Model file for the job. Use its own axes, mm. Round coordinates to 2 decimals unless told otherwise and drop trailing zeros. Loops run counter-clockwise (first coordinate to the right, second up) from the corner with the lowest first, then second, coordinate; pieces in that order, holes last. Notation, with made-up numbers: M 32.25,69 L 50.25,69 A26 cw 50.25,91 Z; hole C 60.25,-6.5 d8. An arc over 180 degrees is marked long. Use a Markdown table: item, result. Add a question column.
Item 1: Saw through at C-C on z = 0.6. Write the cut outline in (x, y).
Item 2: Saw through at B-B on x = 63. Write the cut outline in (y, z).
Item 3: Wall check: L1, parallel to X at y = 52.5, z = 0.1; L2, parallel to Y at x = 63, z = 0.7; L3, parallel to Y at x = -4, z = 0.45. Give the ranges that are in metal, low to high. Write a range as from..to.
Item 4: Saw through at D-D on x = 13. Write the cut outline in (y, z).
Item 5: Saw through at A-A on y = 55. Write the cut outline in (x, z), then the cut area to 3 significant figures.
```python
from build123d import *

# Parameters (mm, degrees)
F0_W     = 136
F0_H     = 120
F1_DEPTH = 1
F2_W     = 116
F2_H     = 10
F3_DEPTH = 1
F4_R     = 1.5
F5_DEPTH = 1


with BuildPart() as f1:
    # F0 (on Top) → F1 (new body)
    with BuildSketch(Plane.XY):
        Rectangle(F0_W, F0_H)
    extrude(amount=F1_DEPTH)

    # F2 (on face) → F3 (cut, through all)
    with BuildSketch(Plane.XY.offset(1)):
        Polygon((58, 60), (-58, 60), (-58, 50), (-45, 50), (-45, 40), (0, 40), (45, 40), (45, 50), (58, 50), align=None)
        with Locations((0, -55)):
            Rectangle(F2_W, F2_H)
    extrude(amount=-F3_DEPTH, mode=Mode.SUBTRACT)

    # F4 (on face) → F5 (cut, through all)
    with BuildSketch(Plane.XY.offset(1)):
        with Locations((-63, 55)):
            Circle(F4_R)
        with Locations((63, 55)):
            Circle(F4_R)
    extrude(amount=-F5_DEPTH, mode=Mode.SUBTRACT)


solid = f1.part
```
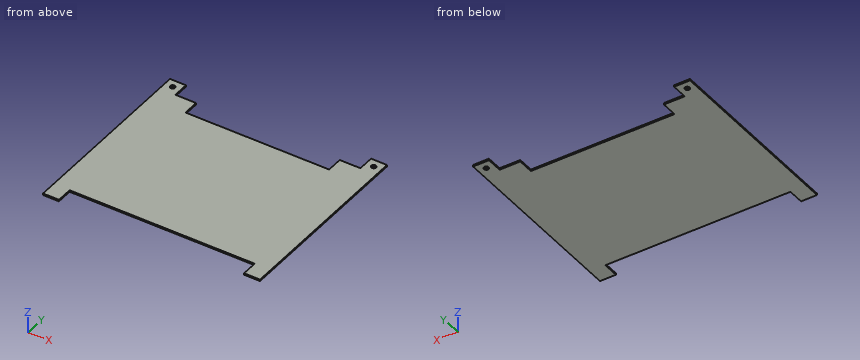
Entries:
| question | item | result |
|---|---|---|
| 1 | outline | M -68,-60 L -58,-60 L -58,-50 L 58,-50 L 58,-60 L 68,-60 L 68,60 L 58,60 L 58,50 L 45,50 L 45,40 L -45,40 L -45,50 L -58,50 L -58,60 L -68,60 Z; hole C -63,55 d3; hole C 63,55 d3 |
| 2 | outline | M -60,0 L 53.5,0 L 53.5,1 L -60,1 Z; M 56.5,0 L 60,0 L 60,1 L 56.5,1 Z |
| 3 | L1 | -68..-58, 58..68 |
| 3 | L2 | -60..53.5, 56.5..60 |
| 3 | L3 | -50..40 |
| 4 | outline | M -50,0 L 40,0 L 40,1 L -50,1 Z |
| 5 | outline | M -68,0 L -64.5,0 L -64.5,1 L -68,1 Z; M -61.5,0 L -58,0 L -58,1 L -61.5,1 Z; M 58,0 L 61.5,0 L 61.5,1 L 58,1 Z; M 64.5,0 L 68,0 L 68,1 L 64.5,1 Z |
| 5 | area | 14.0 mm2 |
